Design review of the part built by this model. Coordinates are the model's own, in mm. A direction names the side the tool comes from. Coordinates: 2 decimals unless noted, no trailing zeros. Loops run counter-clockwise (first coordinate to the right, second up) from the corner with the lowest first, then second, coordinate; pieces in that order, holes last. Notation, with made-up numbers: (-12.75, 23.5) - (38.25, 23.5) arc R18 ccw to (38.25, 57.5) - close; hole circle Ø8 at (85, 85). An arc over 180 degrees is marked (long way). One line per question, with ' | ' between items.
from build123d import *

# Parameters (mm, degrees)
F1_DEPTH = 25.4


with BuildPart() as f1:
    # F0 (on Front) → F1 (new body)
    with BuildSketch(Plane.XZ):
        with BuildLine():
            ThreePointArc((-5.8723054883, -29.3974713107), (-0.0113045982, -25.4959433684), (5.8471949357, -29.4012263195))
            ThreePointArc((5.8471949357, -29.4012263195), (7.8665830511, -33.8356885101), (10.1664885318, -38.131362853))
            ThreePointArc((10.1664885318, -38.131362853), (22.2433688947, -22.2960530681), (38.0304113332, -10.1561450647))
            ThreePointArc((38.0304113332, -10.1561450647), (33.7877497726, -7.8805671775), (29.4089474828, -5.8794369107))
            ThreePointArc((29.4089474828, -5.8794369107), (25.5132673299, -0.0171496036), (29.4195896796, 5.8380516761))
            ThreePointArc((29.4195896796, 5.8380516761), (33.8245563846, 7.8420080033), (38.0926920423, 10.1229268184))
            ThreePointArc((38.0926920423, 10.1229268184), (22.3048159694, 22.2586636554), (10.2296361263, 38.0929041244))
            ThreePointArc((10.2296361263, 38.0929041244), (7.8862120567, 33.7206748888), (5.832770092, 29.2049910031))
            ThreePointArc((5.832770092, 29.2049910031), (-0.0278322356, 25.2936581115), (-5.8914533675, 29.2004639491))
            ThreePointArc((-5.8914533675, 29.2004639491), (-7.8681260767, 33.5542655176), (-10.1128070971, 37.7761407186))
            ThreePointArc((-10.1128070971, 37.7761407186), (-22.1909246105, 22.1248469042), (-37.8860679576, 10.1037655868))
            ThreePointArc((-37.8860679576, 10.1037655868), (-33.7659122536, 7.9077693057), (-29.519257568, 5.9676644959))
            ThreePointArc((-29.519257568, 5.9676644959), (-25.6301816612, 0.0965438971), (-29.5513078142, -5.7532200459))
            ThreePointArc((-29.5513078142, -5.7532200459), (-34.2211473212, -7.8745098641), (-38.736597903, -10.3071992315))
            ThreePointArc((-38.736597903, -10.3071992315), (-22.7195783494, -22.5870715801), (-10.5053141935, -38.6541787064))
            ThreePointArc((-10.5053141935, -38.6541787064), (-8.0309058523, -34.1048564095), (-5.8723054883, -29.3974713107))
        make_face()
        Polygon((15.4941124372, -15.4270198163), (12.5798481763, -17.8831731103), (9.2833515942, -19.7959552386), (5.7047850715, -21.1072472842), (1.9528815413, -21.7772063019), (-1.8583593065, -21.7854759259), (-5.613134847, -21.1318048879), (-9.1973581256, -19.8360546515), (-12.5021243317, -17.9375959321), (-15.4270198163, -15.4941124372), (-17.8831731103, -12.5798481763), (-19.7959552386, -9.2833515942), (-21.1072472842, -5.7047850715), (-21.7772063019, -1.9528815413), (-21.7854759259, 1.8583593065), (-21.1318048879, 5.613134847), (-19.8360546515, 9.1973581256), (-17.9375959321, 12.5021243317), (-15.4941124372, 15.4270198163), (-12.5798481763, 17.8831731103), (-9.2833515942, 19.7959552386), (-5.7047850715, 21.1072472842), (-1.9528815413, 21.7772063019), (1.8583593065, 21.7854759259), (5.613134847, 21.1318048879), (9.1973581256, 19.8360546515), (12.5021243317, 17.9375959321), (15.4270198163, 15.4941124372), (17.8831731103, 12.5798481763), (19.7959552386, 9.2833515942), (21.1072472842, 5.7047850715), (21.7772063019, 1.9528815413), (21.7854759259, -1.8583593065), (21.1318048879, -5.613134847), (19.8360546515, -9.1973581256), (17.9375959321, -12.5021243317), align=None, mode=Mode.SUBTRACT)
        with BuildLine():
            ThreePointArc((38.0304113332, -10.1561450647), (22.2433688947, -22.2960530681), (10.1664885318, -38.131362853))
            ThreePointArc((10.1664885318, -38.131362853), (22.0522532258, -53.6697738876), (37.5164127114, -65.6519853381))
            ThreePointArc((37.5164127114, -65.6519853381), (53.4213887804, -53.5472360443), (65.6235914885, -37.7169022421))
            ThreePointArc((65.6235914885, -37.7169022421), (53.6333778688, -22.1280221412), (38.0304113332, -10.1561450647))
        make_face()
        with BuildLine():
            ThreePointArc((37.5164127114, -65.6519853381), (22.0522532258, -53.6697738876), (10.1664885318, -38.131362853))
            ThreePointArc((10.1664885318, -38.131362853), (3.7508996959, -52.7209861968), (0.5304546679, -68.3301381035))
            ThreePointArc((0.5304546679, -68.3301381035), (2.3669091486, -73.4489662261), (7.4915009075, -75.2692754617))
            ThreePointArc((7.4915009075, -75.2692754617), (23.0077646864, -72.0335045543), (37.5164127114, -65.6519853381))
        make_face()
        with BuildLine():
            ThreePointArc((65.6235914885, -37.7169022421), (53.4213887804, -53.5472360443), (37.5164127114, -65.6519853381))
            ThreePointArc((37.5164127114, -65.6519853381), (52.5012422767, -72.3700363612), (68.5807077231, -75.7059196936))
            ThreePointArc((68.5807077231, -75.7059196936), (73.6678671005, -73.8876561642), (75.5140176195, -68.8105505857))
            ThreePointArc((75.5140176195, -68.8105505857), (72.2649671763, -52.7242023626), (65.6235914885, -37.7169022421))
        make_face()
        with BuildLine():
            ThreePointArc((68.5341561345, -0.3654146815), (52.7586923315, -3.6294921253), (38.0304113332, -10.1561450647))
            ThreePointArc((38.0304113332, -10.1561450647), (53.6333778688, -22.1280221412), (65.6235914885, -37.7169022421))
            ThreePointArc((65.6235914885, -37.7169022421), (72.1596460359, -23.0463732384), (75.4693013087, -7.3304382592))
            ThreePointArc((75.4693013087, -7.3304382592), (73.6519305037, -2.2048036873), (68.5341561345, -0.3654146815))
        make_face()
        with BuildLine():
            ThreePointArc((-1.0124612587, -68.2357638288), (-4.2291126973, -52.9540601379), (-10.5053141935, -38.6541787064))
            ThreePointArc((-10.5053141935, -38.6541787064), (-22.2999024948, -53.8714051532), (-37.5422616312, -65.6334960339))
            ThreePointArc((-37.5422616312, -65.6334960339), (-23.2716891442, -71.9418906098), (-8.0151108309, -75.2102081286))
            ThreePointArc((-8.0151108309, -75.2102081286), (-2.846828708, -73.396684639), (-1.0124612587, -68.2357638288))
        make_face()
        with BuildLine():
            ThreePointArc((-37.5422616312, -65.6334960339), (-22.2999024948, -53.8714051532), (-10.5053141935, -38.6541787064))
            ThreePointArc((-10.5053141935, -38.6541787064), (-22.7195783494, -22.5870715801), (-38.736597903, -10.3071992315))
            ThreePointArc((-38.736597903, -10.3071992315), (-54.0397274181, -22.0854974937), (-65.8642633829, -37.35292793))
            ThreePointArc((-65.8642633829, -37.35292793), (-53.5939421159, -53.3866616113), (-37.5422616312, -65.6334960339))
        make_face()
        with BuildLine():
            ThreePointArc((-69.0824706786, -75.7464577386), (-52.7543029668, -72.4304590644), (-37.5422616312, -65.6334960339))
            ThreePointArc((-37.5422616312, -65.6334960339), (-53.5939421159, -53.3866616113), (-65.8642633829, -37.35292793))
            ThreePointArc((-65.8642633829, -37.35292793), (-72.6638709017, -52.5414311261), (-75.9800079654, -68.8487462552))
            ThreePointArc((-75.9800079654, -68.8487462552), (-74.1461583123, -73.9124802036), (-69.0824706786, -75.7464577386))
        make_face()
        with BuildLine():
            ThreePointArc((-65.8642633829, -37.35292793), (-54.0397274181, -22.0854974937), (-38.736597903, -10.3071992315))
            ThreePointArc((-38.736597903, -10.3071992315), (-56.6892276099, -2.8775463892), (-75.9399100658, -0.249261829))
            ThreePointArc((-75.9399100658, -0.249261829), (-73.2815706098, -19.4472531015), (-65.8642633829, -37.35292793))
        make_face()
        with BuildLine():
            ThreePointArc((10.2296361263, 38.0929041244), (22.3048159694, 22.2586636554), (38.0926920423, 10.1229268184))
            ThreePointArc((38.0926920423, 10.1229268184), (53.8901327799, 22.2426205771), (65.98720102, 38.0573937547))
            ThreePointArc((65.98720102, 38.0573937547), (53.8722995346, 53.8263794302), (38.0568216949, 65.8805242749))
            ThreePointArc((38.0568216949, 65.8805242749), (22.3163343559, 53.8162099791), (10.2296361263, 38.0929041244))
        make_face()
        with BuildLine():
            ThreePointArc((65.98720102, 38.0573937547), (53.8901327799, 22.2426205771), (38.0926920423, 10.1229268184))
            ThreePointArc((38.0926920423, 10.1229268184), (52.9360390158, 3.5663420182), (68.8360344261, 0.3253700086))
            ThreePointArc((68.8360344261, 0.3253700086), (73.9131252899, 2.1506004529), (75.7537769417, 7.2221208671))
            ThreePointArc((75.7537769417, 7.2221208671), (72.5431064158, 23.169531937), (65.98720102, 38.0573937547))
        make_face()
        with BuildLine():
            ThreePointArc((38.0568216949, 65.8805242749), (53.8722995346, 53.8263794302), (65.98720102, 38.0573937547))
            ThreePointArc((65.98720102, 38.0573937547), (72.5131078913, 52.9048408511), (75.7315907831, 68.8006111581))
            ThreePointArc((75.7315907831, 68.8006111581), (73.892228478, 73.884618477), (68.8027604139, 75.7088166387))
            ThreePointArc((68.8027604139, 75.7088166387), (52.9024303983, 72.4444177186), (38.0568216949, 65.8805242749))
        make_face()
        with BuildLine():
            ThreePointArc((0.5764462826, 68.5849581522), (3.7735517842, 52.8230665558), (10.2296361263, 38.0929041244))
            ThreePointArc((10.2296361263, 38.0929041244), (22.3163343559, 53.8162099791), (38.0568216949, 65.8805242749))
            ThreePointArc((38.0568216949, 65.8805242749), (23.2822699561, 72.3357001965), (7.473197141, 75.5027006678))
            ThreePointArc((7.473197141, 75.5027006678), (2.4016767268, 73.662049016), (0.5764462826, 68.5849581522))
        make_face()
        with BuildLine():
            ThreePointArc((-68.7189010029, 0.2348885395), (-52.7728201927, 3.5145237384), (-37.8860679576, 10.1037655868))
            ThreePointArc((-37.8860679576, 10.1037655868), (-53.780428185, 22.2248734645), (-65.9847602554, 38.0554205788))
            ThreePointArc((-65.9847602554, 38.0554205788), (-72.4904161681, 23.1055098819), (-75.6526730835, 7.1110258359))
            ThreePointArc((-75.6526730835, 7.1110258359), (-73.79835158, 2.0468763691), (-68.7189010029, 0.2348885395))
        make_face()
        with BuildLine():
            ThreePointArc((-65.9847602554, 38.0554205788), (-53.780428185, 22.2248734645), (-37.8860679576, 10.1037655868))
            ThreePointArc((-37.8860679576, 10.1037655868), (-22.1909246105, 22.1248469042), (-10.1128070971, 37.7761407186))
            ThreePointArc((-10.1128070971, 37.7761407186), (-22.3186885042, 53.7740285117), (-38.2722920555, 66.0377346602))
            ThreePointArc((-38.2722920555, 66.0377346602), (-53.9753237868, 53.8755657611), (-65.9847602554, 38.0554205788))
        make_face()
        with BuildLine():
            ThreePointArc((-75.9311179626, 68.9827924054), (-72.6216588957, 52.9840480262), (-65.9847602554, 38.0554205788))
            ThreePointArc((-65.9847602554, 38.0554205788), (-53.9753237868, 53.8755657611), (-38.2722920555, 66.0377346602))
            ThreePointArc((-38.2722920555, 66.0377346602), (-53.1019338593, 72.6132353792), (-68.9843197188, 75.9155535265))
            ThreePointArc((-68.9843197188, 75.9155535265), (-74.0964323111, 74.0912044249), (-75.9311179626, 68.9827924054))
        make_face()
        with BuildLine():
            ThreePointArc((-38.2722920555, 66.0377346602), (-22.3186885042, 53.7740285117), (-10.1128070971, 37.7761407186))
            ThreePointArc((-10.1128070971, 37.7761407186), (-3.3821811813, 52.9097624233), (-0.077326994, 69.1395427644))
            ThreePointArc((-0.077326994, 69.1395427644), (-1.9087320963, 74.2120247418), (-6.9799378863, 76.0469606796))
            ThreePointArc((-6.9799378863, 76.0469606796), (-23.1742648581, 72.7560566396), (-38.2722920555, 66.0377346602))
        make_face()
    extrude(amount=F1_DEPTH)


solid = f1.part
Q1. Take a section at A-A (z = 45). Give the boundary of the cut face in (x, y), plus the area to 3 significant figures.
Returned:
outline: (-69.55, -25.4) - (-6.41, -25.4) - (-6.41, 0) - (-69.55, 0) - close; (6.74, -25.4) - (69.51, -25.4) - (69.51, 0) - (6.74, 0) - close | area: 3,200 mm²
Q2. For pin 1 (4 mm diameter, centred on x = -12.5, y = -16.5, fed in from +Z); pin 2 (12 mm diameter, centred on x = 47.5, y = -20, fed in from +Z); pin 3 (12 mm diameter, centred on y = -19, z = 9, fed in from -X), all flat-tipped, find the tip position at first contact; note any pin that passes through.
Returned:
pin 1: stops at z = 75.64 | pin 2: stops at z = 72.63 | pin 3: stops at x = -75.68
Q3. Take a section at B-B (x = -54.5). Give the boundary of the cut face in (y, z), plus the area to 3 significant figures.
Returned:
outline: (-25.4, -72.97) - (0, -72.97) - (0, -3.5) - (-25.4, -3.5) - close; (-25.4, 2.98) - (0, 2.98) - (0, 73.05) - (-25.4, 73.05) - close | area: 3,540 mm²
Q4. Tool access review of faces 4 (the cylindrical face through (-72.422, -12.522, 23.324)), 5 (the cylindrical face through (-7.839, -12.522, 33.494)): name each direction out of +Z, -Z, +X, -X, +Y, -Y from which nothing blocks a thin tool from reaching the whole face with its end or side.
Returned:
face 4: -X, +Y, -Y | face 5: +Y, -Y
Q5. Draft analysis for pull direction Z (two halves, no side actions). For faces 1 (the flat face through (18.8, -12.5, 11)), 2 (the cylindrical face through (-52.885, -12.522, 72.543)), 3 (the flat face through (16, 0, 18)), state which applies: +Z half, -Z half, draft (parallel to the pull), parting line (faces both ways), or undercut.
Returned:
face 1: undercut | face 2: +Z half | face 3: draft
Q6. To check wall thickness, follow line 1 along X through (y, z) = (-18.75, 16.5); line 2 along X through (y, z) = (-14, -50); line 3 along Z through (x, y) = (14.5, -16.25). State the ranges of each line that lie inside material, in increasing order.
Returned:
line 1: x = -74.23 to -14.22, 14.22 to 74.32 | line 2: x = -71.8 to -5.24, 4.68 to 71.34 | line 3: z = -74.23 to -16.26, 16.27 to 74.53
